Build history of the part. All positions in model axes, mm. Face numbers are marked on the shaded views. A direction names the side the tool comes from. Coordinates: 2 decimals unless noted, no trailing zeros. Order: outer loops, then holes, each group sorted by start corner. A loop starts at its lowest first (then second) coordinate and runs counter-clockwise, first axis right, second up. Notation, with made-up numbers: M 76.5,-38 L 116.5,-38 A23 cw 116.5,1 Z; hole C 51.5,39 d4. An arc over 180 degrees is marked long. Write item = value, one per line. Start each with the question number.
Q1. 3-axis set-ups, long thin cutter, end or side, ignore diameter. For the marked faces 4, 5 and 6: which of +Z, -Z, +X, -X, +Y, -Y reach the whole face in a straight line?
Q2. Band-saw the part on A-A on y = 3.5. Write the cut outline in (x, z).
Q3. Drill centre lines: probe 1 along Y at (x, z) = (-0.25, 6.75); probe 2 along Y at (x, z) = (2, 4.75); probe 3 along X at (y, z) = (-2.5, 17.5). Where is each one in solid material? Low to high.
Q4. Pull direction X, two halves, no side cores. Call the marked faces 1, 2 and 3: released by +X, released by -X, zero draft, split by the parting line, or undercut.
Q5. Pin check, flat tips, straight feed: P1, Ø1.5, axis at x = 4, z = 16.5, coming from the -Y side; P2, Ø4, axis at y = -1.5, z = 11, coming from the +X side; P3, Ø1, axis at x = -7.5, z = 6, coming from the -Y side; P4, Ø1.5, axis at y = 3.5, z = 12.5, coming from the +X side. Stop position of each tip, or through.
```python
from build123d import *

# Parameters (mm, degrees)
PAD_DEPTH   = 25
FILLET_R    = 1
FILLET001_R = 7.8
FILLET002_R = 2
FILLET003_R = 0.25


with BuildPart() as part:
    # Sketch → Pad (new body)
    with BuildSketch(Plane.XY):
        with BuildLine():
            Line((-1.8, 5), (-3.414214, 5))
            Line((-3.414214, 5), (-4.207107, 4.207107))
            ThreePointArc((-4.207107, 4.207107), (-4.42388, 3.117317), (-3.5, 2.5))
            Line((-3.5, 2.5), (-3, 2.5))
            Line((-3, 2.5), (-3, 0))
            Line((-3, 0), (-10, 0))
            Line((-10, 0), (-8.556624, -2.5))
            Line((-8.556624, -2.5), (-8.556624, -7.5))
            Line((-8.556624, -7.5), (8.556624, -7.5))
            Line((8.556624, -7.5), (8.556624, -2.5))
            Line((8.556624, -2.5), (10, 0))
            Line((10, 0), (3, 0))
            Line((3, 0), (3, 2.5))
            Line((3, 2.5), (3.5, 2.5))
            ThreePointArc((3.5, 2.5), (4.42388, 3.117317), (4.207107, 4.207107))
            Line((4.207107, 4.207107), (3.414214, 5))
            Line((3.414214, 5), (1.8, 5))
            Line((1.8, 5), (1.8, -1.2))
            Line((1.8, -1.2), (7.317787, -1.2))
            ThreePointArc((-7.317787, -1.2), (0, -6.3), (7.317787, -1.2))
            Line((-7.317787, -1.2), (-1.8, -1.2))
            Line((-1.8, -1.2), (-1.8, 5))
        make_face()
    extrude(amount=PAD_DEPTH)

    # Fillet
    fillet_edges = [part.edges().sort_by_distance(p)[0] for p in [
        (-8.556624, -2.5, 12.5),
        (8.556624, -2.5, 12.5),
        (10, 0, 12.5),
        (-10, 0, 12.5),
        (7.317787, -1.2, 12.5),
        (-7.317787, -1.2, 12.5),
        (1.8, -1.2, 12.5),
        (-1.8, -1.2, 12.5),
        (3, 0, 12.5),
        (-3, 0, 12.5),
        (3, 2.5, 12.5),
        (-3, 2.5, 12.5),
    ]]
    fillet(fillet_edges, radius=FILLET_R)

    # Fillet001
    fillet001_edges = [part.edges().sort_by_distance(p)[0] for p in [
        (-8.556624, -7.5, 12.5),
        (8.556624, -7.5, 12.5),
    ]]
    fillet(fillet001_edges, radius=FILLET001_R)

    # Fillet002
    fillet002_edges = [part.edges().sort_by_distance(p)[0] for p in [
        (-3.414214, 5, 12.5),
        (3.414214, 5, 12.5),
    ]]
    fillet(fillet002_edges, radius=FILLET002_R)

    # Fillet003
    fillet003_edges = [part.edges().sort_by_distance(p)[0] for p in [
        (-1.8, 5, 12.5),
        (1.8, 5, 12.5),
    ]]
    fillet(fillet003_edges, radius=FILLET003_R)


solid = part.part
```
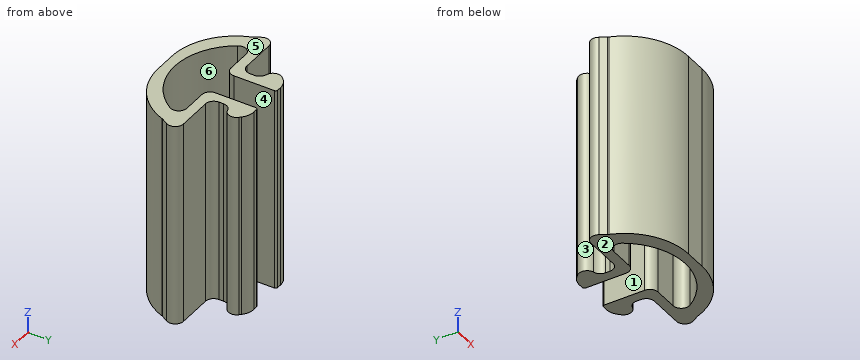
Recorded:
q1.face_4 = +Z, -Z, +Y
q1.face_5 = +Z, +X, -X, +Y, -Y
q1.face_6 = +Z, -Z
q2.outline = M -4.5,0 L -1.8,0 L -1.8,25 L -4.5,25 Z; M 1.8,0 L 4.5,0 L 4.5,25 L 1.8,25 Z
q3.probe_1 = -7.5 to -6.3
q3.probe_2 = -7.47 to -6.04, -0.8 to 4.99
q3.probe_3 = -8.59 to -6.66, 6.66 to 8.59
q4.face_1 = undercut
q4.face_2 = zero draft
q4.face_3 = released by -X
q5.P1 = -7.25
q5.P2 = 9.27
q5.P3 = -5.03
q5.P4 = 4.5
